Can you work these out from the drawing? Everything is in mm from the part's minimum corner. Coordinates: 2 decimals unless noted, no trailing zeros. Loops run counter-clockwise (first coordinate to the right, second up) from the corner with the lowest first, then second, coordinate; pieces in that order, holes last.
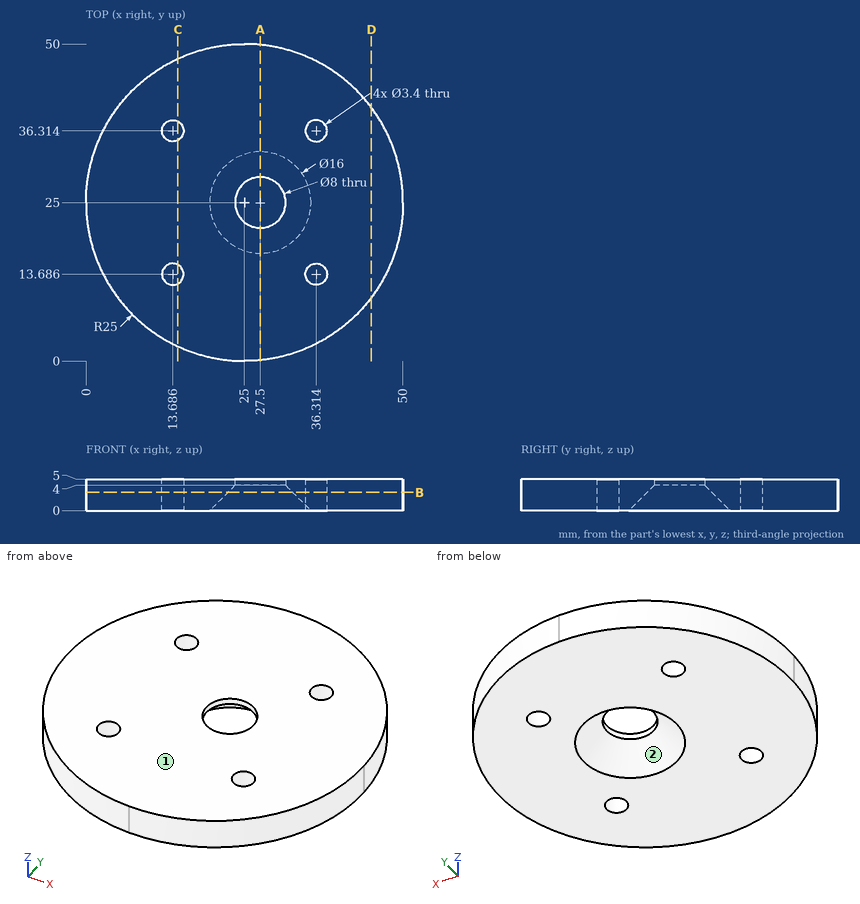
1) We'd pull the mould along X, two halves only. Please class the marked faces 1 and 2: released by +X, released by -X, zero draft, split by the parting line, or undercut.
2) Imagine slicing it at C-C on x = 14.5. List the corners of the cut face in (y, z) for me.
3) Imagine slicing it at D-D on x = 45. List the corners of the cut face in (y, z) for me, plus the area to 3 significant figures.
4) If I drill on L1, parallel to Y at x = 15, z = 2.2 (1 decimal); L2, parallel to Y at x = 35.5, z = 1.85; L3, parallel to X at y = 13.5, z = 2.3 (1 decimal), over which ranges is the centre line in solid material (lowest first)?
5) Will these pins go through, and if not, where does the flat tip stop? pin 1 (3 mm diameter, centred on x = 15, z = 3.5, fed in from +Y); pin 2 (1 mm diameter, centred on x = 41, z = 2, fed in from +Y) (1 decimal); pin 3 (3 mm diameter, centred on x = 36.5, z = 2, fed in from +Y).
6) Imagine slicing it at A-A on x = 27.5. List the corners of the cut face in (y, z) for me (1 decimal), plus the area to 3 significant figures.
7) Imagine slicing it at B-B on z = 2.9. List the corners of the cut face in (x, y) for me.
Solved:
1. face 1: zero draft
1. face 2: undercut
2. outline: (2.31, 0) - (12.19, 0) - (12.19, 5) - (2.31, 5) - close; (15.18, 0) - (34.82, 0) - (34.82, 5) - (15.18, 5) - close; (37.81, 0) - (47.69, 0) - (47.69, 5) - (37.81, 5) - close
3. outline: (10, 0) - (40, 0) - (40, 5) - (10, 5) - close
3. area: 150 mm2
4. L1: y = 2.1 to 12.6, 14.8 to 35.2, 37.4 to 47.9
4. L2: y = 2.31 to 12.19, 15.18 to 34.82, 37.81 to 47.69
4. L3: x = 2.8 to 12, 15.4 to 34.6, 38 to 47.2
5. pin 1: stops at y = 48.51
5. pin 2: stops at y = 44.6
5. pin 3: stops at y = 47.91
6. outline: (0.1, 0) - (17, 0) - (21, 4) - (21, 5) - (0.1, 5) - close; (29, 4) - (33, 0) - (49.9, 0) - (49.9, 5) - (29, 5) - close
6. area: 193 mm2
7. outline: (0, 25) arc R25 ccw to (25, 0) arc R25 ccw to (50, 25) arc R25 ccw to (25, 50) arc R25 ccw to start; hole circle Ø3.4 at (13.69, 13.69); hole circle Ø3.4 at (13.69, 36.31); hole circle Ø10.2 at (27.5, 25); hole circle Ø3.4 at (36.31, 13.69); hole circle Ø3.4 at (36.31, 36.31)
